Can you work these out from the model? Positions are in its coordinate system, mm. A direction names the side the tool comes from. Coordinates: 2 decimals unless noted, no trailing zeros. Put each result on its own line as item: value. Start each with the question number.
from build123d import *

# Parameters (mm, degrees)
SKETCH_1_W              = 6.4
SKETCH_1_H              = 11
EXTRUDE_1_DEPTH         = 3.678333878
FILLET_1_R              = 3.2
EXTRUDE_2_DEPTH         = 1.5
SKETCH_3_W              = 4.04000003
SKETCH_3_H              = 1.2
CUT_EXTRUDE_1_DEPTH     = 0.5
FILLET_2_R              = 0.25
FILLET_3_R              = 0.2
OTHER_2_OUTLINE_W       = 1.5
OTHER_2_OUTLINE_H       = 1.5
OTHER_2_DEPTH           = 2
SKETCH_5_W              = 1.8
SKETCH_5_H              = 1.8
CUT_EXTRUDE_2_DEPTH     = 5.4
CUT_EXTRUDE_START       = -0.1
CUT_EXTRUDE_3_OUTLINE_W = 10
CUT_EXTRUDE_3_OUTLINE_H = 14
CUT_EXTRUDE_3_DEPTH     = 0.1
CHAMFER_1_SIZE          = 0.8


# Read off the part's stored shape, not the designer's step: 压凹2, 切除-拉伸3
# Some blends are built 0.0001 mm under size
with BuildPart() as part:
    # 草图1 → 凸台-拉伸1 (new body)
    with BuildSketch(Plane(origin=(0, 0, 0), x_dir=(1, 0, 0), z_dir=(0, 1, 0))):
        Rectangle(SKETCH_1_W, SKETCH_1_H)
    extrude(amount=EXTRUDE_1_DEPTH)

    # 圆角1
    fillet_1_edges = [part.edges().sort_by_distance(p)[0] for p in [
        (-3.2, 1.839166939, -5.5),
        (3.2, 1.839166939, -5.5),
        (3.2, 1.839166939, 5.5),
        (-3.2, 1.839166939, 5.5),
    ]]
    fillet(fillet_1_edges, radius=FILLET_1_R - 0.0001)  # a hair under: the kernel refuses the full size

    # 草图2 → 凸台-拉伸2 (add)
    with BuildSketch(Plane(origin=(0, 3.678333878, 0), x_dir=(1, 0, 0), z_dir=(0, 1, 0))):
        with BuildLine():
            Line((2.020000015, 1), (2.020000015, -0.5))
            ThreePointArc((2.020000015, -0.5), (0, -2.520000015), (-2.020000015, -0.5))
            Line((-2.020000015, -0.5), (-2.020000015, 1))
            ThreePointArc((-2.020000015, 1), (1.5e-08, 3.02), (2.020000015, 1))
        make_face()
    extrude(amount=EXTRUDE_2_DEPTH)

    # 草图3 → 切除-拉伸1 (cut)
    with BuildSketch(Plane(origin=(0, 5.178333878, 0), x_dir=(1, 0, 0), z_dir=(0, 1, 0))):
        with Locations((0, 0.25)):
            Rectangle(SKETCH_3_W, SKETCH_3_H)
    extrude(amount=-CUT_EXTRUDE_1_DEPTH, mode=Mode.SUBTRACT)

    # 圆角2
    # the kernel refuses this fillet: 0.25 mm, written as the material it takes off along each edge
    with BuildSketch(Plane(origin=(2.020000015, 5.838693877, 0.35), x_dir=(-0.012214651008913897, 0, 0.9999253983676635), z_dir=(0, -1, 0))) as fillet_2_piece_1:
        with BuildLine():
            CenterArc((0.253069545, 0.249754592), FILLET_2_R, 179.300134646, 93.238774214)
            Line((0.003088195, 0.252808255), (-0.02190994, 0.253113621))
            Line((-0.02190994, 0.253113621), (-0.024998135, 0.000305366))
            Line((-0.024998135, 0.000305366), (-0.000305366, -0.024998135))
            ThreePointArc((-0.000305366, -0.024998135), (0.149683443, -0.026830333), (0.265251445, -0.024975459))
            Line((0.265251445, -0.024975459), (0.264143999, 0))
        make_face()
    extrude(amount=1.160359998, mode=Mode.SUBTRACT)
    with BuildSketch(Plane(origin=(2.020000015, 5.838693882, -0.85), x_dir=(-0.012214654567378504, 0, -0.9999253983241949), z_dir=(0, -1, 0))) as fillet_2_piece_2:
        with BuildLine():
            CenterArc((0.253069545, -0.249754592), FILLET_2_R, 87.46109086, 93.238774699)
            Line((0.003088196, -0.252808256), (-0.021909939, -0.253113622))
            Line((-0.021909939, -0.253113622), (-0.024998135, -0.000305366))
            Line((-0.024998135, -0.000305366), (-0.000305366, 0.024998135))
            ThreePointArc((-0.000305366, 0.024998135), (0.149683444, 0.026830333), (0.265251447, 0.024975459))
            Line((0.265251447, 0.024975459), (0.264144001, 0))
        make_face()
    extrude(amount=1.160360003, mode=Mode.SUBTRACT)
    with BuildSketch(Plane(origin=(-2.020000015, 5.838693877, 0.35), x_dir=(0.012214651008913804, 0, 0.9999253983676635), z_dir=(0, -1, 0))) as fillet_2_piece_3:
        with BuildLine():
            CenterArc((0.253069545, -0.249754592), FILLET_2_R, 87.461091141, 93.238774214)
            Line((0.003088195, -0.252808255), (-0.02190994, -0.253113621))
            Line((-0.02190994, -0.253113621), (-0.024998135, -0.000305366))
            Line((-0.024998135, -0.000305366), (-0.000305366, 0.024998135))
            ThreePointArc((-0.000305366, 0.024998135), (0.149683443, 0.026830333), (0.265251445, 0.024975459))
            Line((0.265251445, 0.024975459), (0.264143999, 0))
        make_face()
    extrude(amount=1.160359998, mode=Mode.SUBTRACT)
    with BuildSketch(Plane(origin=(-2.020000015, 5.838693882, -0.85), x_dir=(0.012214654567376798, 0, -0.9999253983241947), z_dir=(0, -1, 0))) as fillet_2_piece_4:
        with BuildLine():
            CenterArc((0.253069545, 0.249754592), FILLET_2_R, 179.300134442, 93.238774699)
            Line((0.003088196, 0.252808256), (-0.021909939, 0.253113622))
            Line((-0.021909939, 0.253113622), (-0.024998135, 0.000305366))
            Line((-0.024998135, 0.000305366), (-0.000305366, -0.024998135))
            ThreePointArc((-0.000305366, -0.024998135), (0.149683444, -0.026830333), (0.265251447, -0.024975459))
            Line((0.265251447, -0.024975459), (0.264144001, 0))
        make_face()
    extrude(amount=1.160360003, mode=Mode.SUBTRACT)

    # 圆角3
    fillet_3_edges = [part.edges().sort_by_distance(p)[0] for p in [
        (0, 5.178333878, 2.520000015),
        (0, 5.178333878, 0.35),
        (-1.948874678, 5.178333878, 0.428289595),
        (1.948874678, 5.178333878, 0.428289595),
        (0, 5.178333878, -0.85),
        (0, 5.178333878, -3.02),
        (-1.948874678, 5.178333878, -0.928289595),
        (1.948874678, 5.178333878, -0.928289595),
    ]]
    fillet(fillet_3_edges, radius=FILLET_3_R)

    # 压凹2 outline → 压凹2 (cut)
    with BuildSketch(Plane(origin=(0, 0, 0), x_dir=(1, 0, 0), z_dir=(0, 1, 0))):
        with Locations((0, 1)):
            Rectangle(OTHER_2_OUTLINE_W, OTHER_2_OUTLINE_H)
    extrude(amount=OTHER_2_DEPTH, mode=Mode.SUBTRACT)

    # 草图5 → 切除-拉伸2 (cut)
    with BuildSketch(Plane.XZ.offset(-2)):
        with Locations((0, -1)):
            Rectangle(SKETCH_5_W, SKETCH_5_H)
    extrude(amount=CUT_EXTRUDE_2_DEPTH, mode=Mode.SUBTRACT)

    # 切除-拉伸3 outline → 切除-拉伸3 (cut)
    with BuildSketch(Plane.XZ.offset(CUT_EXTRUDE_START)):
        Rectangle(CUT_EXTRUDE_3_OUTLINE_W, CUT_EXTRUDE_3_OUTLINE_H)
    extrude(amount=CUT_EXTRUDE_3_DEPTH, mode=Mode.SUBTRACT)

    # 倒角1
    chamfer_1_edges = [part.edges().sort_by_distance(p)[0] for p in [
        (2.262770989, 0.1, 4.562770989),
        (-2.262770989, 0.1, -4.562770989),
        (-2.262770989, 0.1, 4.562770989),
        (3.2, 0.1, 0),
        (2.262770989, 0.1, -4.562770989),
        (-3.2, 0.1, 0),
    ]]
    chamfer(chamfer_1_edges, length=CHAMFER_1_SIZE)


solid = part.part
Q1. Please list where these lines run through material, in increasing order: line 1 along Y through (x, z) = (-0.5, -4.25); line 2 along X through (y, z) = (4.2, 0.25); line 3 along Y through (x, z) = (0.75, 0). Write a range as [from, to].
Q2. We'd pull the mould along Z, two halves only. Please class faces 6 (the cylindrical face through (-2.288, 2.309, -4.538)), 7 (the flat face through (-0.9, 1, -1)), 8 (the flat face through (0, 5.178, -2)): released by +Z, released by -Z, zero draft, split by the parting line, or undercut.
Q3. On a 3-axis mill with a long thin cutter (end or side, diameter ignored), from which of +Z, -Z, +X, -X, +Y, -Y can I reach the whole of each face in a straight line? I mean faces 1 (the flat face through (-2.2, 3.678, -0.1)), 2 (the flat face through (2.02, 4, 0)), 3 (the cylindrical face through (-0.04, 4.32, -3.02)), 4 (the flat face through (0, 1, -0.1)), 5 (the conical face through (-1.83, 0.317, -4.17)). Say none if no direction works.
Q4. Will these pins go through, and if not, where does the flat tip stop? pin 1 (0.5 mm diameter, centred on x = -0.5, y = 1.5, fed in from -Z); pin 2 (1 mm diameter, centred on y = 3, z = -3.5, fed in from +X); pin 3 (0.5 mm diameter, centred on x = 0, z = 0, fed in from +Y).
Calculated:
1. line 1: [0.1, 3.68]
1. line 2: [-2.02, 2.02]
1. line 3: [0.1, 4.68]
2. face 6: released by -Z
2. face 7: undercut
2. face 8: zero draft
3. face 1: +Y
3. face 2: +Z, -Z, +X, +Y
3. face 3: -Z, +Y
3. face 4: -Y
3. face 5: -Z, -X, -Y
4. pin 1: z = -5.49
4. pin 2: x = 3.12
4. pin 3: y = 4.68
